Input: part model. Units: mm. Frame: model coordinates. A direction names the side the tool comes from. Coordinates: 2 decimals unless noted, no trailing zeros. Loops run counter-clockwise (first coordinate to the right, second up) from the corner with the lowest first, then second, coordinate; pieces in that order, holes last. Notation, with made-up numbers: (57, -28.75) - (63, -28.75) arc R36 cw to (63, 10.25) - close; hole circle Ø4 at (-17.75, 22.5). An arc over 180 degrees is marked (long way). Use a Markdown table: item, result. Add a question column.
1. Contact query for flat-ended pins moving along their axis: P1, Ø3, axis at y = 22.5, z = 1.5, coming from the +X side; P2, Ø6, axis at x = -1, y = 22, coming from the -Z side; P3, Ø1.5, axis at y = 9.5, z = 3, coming from the +X side; P4, Ø3, axis at x = -3, y = 7.5, coming from the +Z side. Output: stop coordinate, or through.
2. Section query D-D on y = 36.5. Return the cut outline in (x, z) (3 decimals), then the cut area to 3 significant figures.
3. Section query B-B on x = 0. Return the cut outline in (y, z) (3 decimals).
4. Access query for faces 1 (the face through (0, 0, 0)), 2 (the face through (1.78, 36.54, 5.65)). Directions: +Z, -Z, +X, -X, +Y, -Y. A direction counts if a zero-diameter tool reaches every point of the face in a straight line with its end or side. Return the directions, or none.
5. Section query C-C on y = 9. Return the cut outline in (x, z).
6. Ray query, L1, parallel to Y at x = -1.25, z = -1.75; L2, parallel to X at y = 42, z = 2.5; L3, parallel to Z at x = 0.25, y = 36. Return the intervals inside material, ascending. Write a range as [from, to].
7. Section query A-A on z = 0. Return the cut outline in (x, y) (3 decimals).
```python
from build123d import *

# Parameters (mm, degrees)
SKETCH_1_R      = 2
EXTRUDE_1_DEPTH = 35
SKETCH_2_R      = 5.925
EXTRUDE_2_DEPTH = 3
SKETCH_3_R      = 6.25
EXTRUDE_3_DEPTH = 9.5
CHAMFER_1_SIZE  = 4
CHAMFER_1_SIZE2 = 2.309401077
CHAMFER_2_SIZE  = 0.2
CHAMFER_2_SIZE2 = 0.115470054


with BuildPart() as part:
    # 草图1 → 凸台-拉伸1 (new body)
    with BuildSketch(Plane(origin=(0, 0, 0), x_dir=(1, 0, 0), z_dir=(0, 1, 0))):
        with Locations(Location((0, 0, 0), (0, 0, 270))):
            Circle(SKETCH_1_R)
    extrude(amount=EXTRUDE_1_DEPTH)

    # 草图2 → 凸台-拉伸2 (add)
    with BuildSketch(Plane(origin=(0, 35, 0), x_dir=(1, 0, 0), z_dir=(0, 1, 0))):
        with Locations(Location((0, 0, 0), (0, 0, 270))):
            Circle(SKETCH_2_R)
    extrude(amount=EXTRUDE_2_DEPTH)

    # 草图3 → 凸台-拉伸3 (add)
    with BuildSketch(Plane(origin=(0, 38, 0), x_dir=(1, 0, 0), z_dir=(0, 1, 0))):
        with Locations(Location((0, 0, 0), (0, 0, 270))):
            Circle(SKETCH_3_R)
    extrude(amount=EXTRUDE_3_DEPTH)

    # 倒角1
    chamfer_1_edges = [part.edges().sort_by_distance(p)[0] for p in [
        (0, 47.5, -6.25),
    ]]
    chamfer_1_side = [part.faces().sort_by_distance(p)[0] for p in [
        (0, 42.75, -6.25),
    ]]
    chamfer(chamfer_1_edges, length=CHAMFER_1_SIZE, length2=CHAMFER_1_SIZE2, reference=chamfer_1_side[0])

    # 倒角2
    chamfer_2_edges = [part.edges().sort_by_distance(p)[0] for p in [
        (0, 35, -5.925),
    ]]
    chamfer_2_side = [part.faces().sort_by_distance(p)[0] for p in [
        (0, 35, -5.757415693),
    ]]
    chamfer(chamfer_2_edges, length=CHAMFER_2_SIZE, length2=CHAMFER_2_SIZE2, reference=chamfer_2_side[0])


solid = part.part
```
Resolved:
| question | item | result |
|---|---|---|
| 1 | P1 | x = 2 |
| 1 | P2 | z = -2 |
| 1 | P3 | through |
| 1 | P4 | z = 1.32 |
| 2 | outline | circle Ø11.85 at (0, 0) |
| 2 | area | 110 mm² |
| 3 | outline | (0, -2) - (35, -2) - (35, -5.725) - (35.115, -5.925) - (38, -5.925) - (38, -6.25) - (43.5, -6.25) - (47.5, -3.941) - (47.5, 3.941) - (43.5, 6.25) - (38, 6.25) - (38, 5.925) - (35.115, 5.925) - (35, 5.725) - (35, 2) - (0, 2) - close |
| 4 | face 1 | +Z, -Z, +X, -X, -Y |
| 4 | face 2 | -Y |
| 5 | outline | circle Ø4 at (0, 0) |
| 6 | L1 | [35, 47.5] |
| 6 | L2 | [-5.73, 5.73] |
| 6 | L3 | [-5.92, 5.92] |
| 7 | outline | (-6.25, 38) - (-5.925, 38) - (-5.925, 35.115) - (-5.725, 35) - (-2, 35) - (-2, 0) - (2, 0) - (2, 35) - (5.725, 35) - (5.925, 35.115) - (5.925, 38) - (6.25, 38) - (6.25, 43.5) - (3.941, 47.5) - (-3.941, 47.5) - (-6.25, 43.5) - close |
